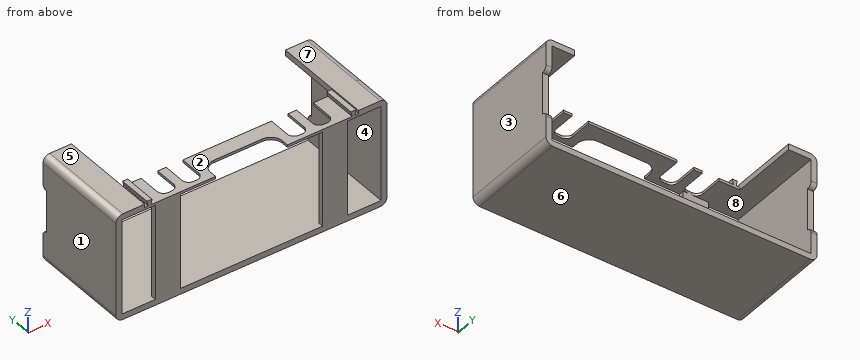
```python
from build123d import *

# Parameters (mm, degrees)
SKETCH1_W           = 81
SKETCH1_H           = 32
BOSS_EXTRUDE1_DEPTH = 10
SKETCH2_W           = 77.5
SKETCH2_H           = 28.5
CUT_EXTRUDE1_DEPTH  = 10
SKETCH3_W           = 7.5
SKETCH3_H           = 32
BOSS_EXTRUDE2_DEPTH = 1.5
SKETCH4_W           = 64
SKETCH4_H           = 1
CUT_EXTRUDE2_DEPTH  = 10
BOSS_EXTRUDE3_DEPTH = 10
BOSS_EXTRUDE4_DEPTH = 10
FILLET1_R           = 2
FILLET2_R           = 2
FILLET3_R           = 2
FILLET4_R           = 2
CUT_EXTRUDE3_DEPTH  = 0.75
SKETCH8_W           = 21.5
SKETCH8_H           = 5.5
CUT_EXTRUDE4_DEPTH  = 0.75
FILLET5_R           = 3.5
FILLET6_R           = 3.5
BOSS_EXTRUDE5_START = 20
BOSS_EXTRUDE5_DEPTH = 20
SKETCH10_W          = 1.75
SKETCH10_H          = 12.5
CUT_EXTRUDE5_DEPTH  = 1.5
FILLET7_R           = 1.5
FILLET8_R           = 1.5
FILLET10_R          = 1.5
FILLET11_R          = 1.5


with BuildPart() as part:
    # Sketch1 → Boss-Extrude1 (new body)
    with BuildSketch(Plane(origin=(0, 0, 0), x_dir=(1, 0, 0), z_dir=(0, 1, 0))):
        with Locations((-86.056207425, -60.23876691)):
            Rectangle(SKETCH1_W, SKETCH1_H)
    extrude(amount=BOSS_EXTRUDE1_DEPTH)

    # Sketch2 → Cut-Extrude1 (cut)
    with BuildSketch(Plane(origin=(0, 10, 0), x_dir=(1, 0, 0), z_dir=(0, 1, 0))):
        with Locations((-86.056207425, -60.23876691)):
            Rectangle(SKETCH2_W, SKETCH2_H)
    extrude(amount=-CUT_EXTRUDE1_DEPTH, mode=Mode.SUBTRACT)

    # Sketch3 → Boss-Extrude2 (add)
    with BuildSketch(Plane(origin=(0, 0, 0), x_dir=(-1, 0, 0), z_dir=(0, -1, 0))):
        with Locations((61.056207425, -60.23876691)):
            Rectangle(SKETCH3_W, SKETCH3_H)
        with Locations((111.056207425, -60.23876691)):
            Rectangle(SKETCH3_W, SKETCH3_H)
    extrude(amount=-BOSS_EXTRUDE2_DEPTH)

    # Sketch4 → Cut-Extrude2 (cut)
    with BuildSketch(Plane(origin=(0, 10, 0), x_dir=(1, 0, 0), z_dir=(0, 1, 0))):
        with Locations((-86.056207425, -75.73876691)):
            Rectangle(SKETCH4_W, SKETCH4_H)
    extrude(amount=-CUT_EXTRUDE2_DEPTH, mode=Mode.SUBTRACT)

    # Sketch5 → Boss-Extrude3 (add)
    with BuildSketch(Plane(origin=(0, 10, 0), x_dir=(1, 0, 0), z_dir=(0, 1, 0))):
        Polygon((-116.976207425, -75.23876691), (-117.306207425, -76.781751031), (-115.806207425, -76.781751031), (-116.146207425, -75.23876691), align=None)
    extrude(amount=-BOSS_EXTRUDE3_DEPTH)

    # Sketch6 → Boss-Extrude4 (add)
    with BuildSketch(Plane(origin=(0, 10, 0), x_dir=(1, 0, 0), z_dir=(0, 1, 0))):
        Polygon((-55.966207425, -75.23876691), (-56.306207425, -76.781751031), (-54.806207425, -76.781751031), (-55.136207425, -75.23876691), align=None)
    extrude(amount=-BOSS_EXTRUDE4_DEPTH)

    # Fillet1
    fillet1_edges = [part.edges().sort_by_distance(p)[0] for p in [
        (-126.556207425, 5, 76.23876691),
    ]]
    fillet(fillet1_edges, radius=FILLET1_R)

    # Fillet2
    fillet2_edges = [part.edges().sort_by_distance(p)[0] for p in [
        (-45.556207425, 5, 76.23876691),
    ]]
    fillet(fillet2_edges, radius=FILLET2_R)

    # Fillet3
    fillet3_edges = [part.edges().sort_by_distance(p)[0] for p in [
        (-45.556207425, 5, 44.23876691),
    ]]
    fillet(fillet3_edges, radius=FILLET3_R)

    # Fillet4
    fillet4_edges = [part.edges().sort_by_distance(p)[0] for p in [
        (-126.556207425, 5, 44.23876691),
    ]]
    fillet(fillet4_edges, radius=FILLET4_R)

    # Sketch7 → Cut-Extrude3 (cut)
    with BuildSketch(Plane.XY.offset(75.23876691)):
        with BuildLine():
            Line((-111.806207425, 10), (-106.806207425, 10))
            Line((-106.806207425, 10), (-106.806207425, 3.5))
            ThreePointArc((-106.806207425, 3.5), (-107.391993862, 2.085786438), (-108.806207425, 1.5))
            Line((-108.806207425, 1.5), (-109.806207425, 1.5))
            ThreePointArc((-109.806207425, 1.5), (-111.220420987, 2.085786438), (-111.806207425, 3.5))
            Line((-111.806207425, 3.5), (-111.806207425, 10))
        make_face()
        with BuildLine():
            Line((-65.306207425, 10), (-60.306207425, 10))
            Line((-60.306207425, 10), (-60.306207425, 3.5))
            ThreePointArc((-60.306207425, 3.5), (-60.891993862, 2.085786438), (-62.306207425, 1.5))
            Line((-62.306207425, 1.5), (-63.306207425, 1.5))
            ThreePointArc((-63.306207425, 1.5), (-64.720420987, 2.085786438), (-65.306207425, 3.5))
            Line((-65.306207425, 3.5), (-65.306207425, 10))
        make_face()
        with BuildLine():
            Line((-104.306207425, 10), (-99.306207425, 10))
            Line((-99.306207425, 10), (-99.306207425, 3.5))
            ThreePointArc((-99.306207425, 3.5), (-99.891993862, 2.085786438), (-101.306207425, 1.5))
            Line((-101.306207425, 1.5), (-102.306207425, 1.5))
            ThreePointArc((-102.306207425, 1.5), (-103.720420987, 2.085786438), (-104.306207425, 3.5))
            Line((-104.306207425, 3.5), (-104.306207425, 10))
        make_face()
        with BuildLine():
            Line((-72.806207425, 10), (-67.806207425, 10))
            Line((-67.806207425, 10), (-67.806207425, 3.5))
            ThreePointArc((-67.806207425, 3.5), (-68.391993862, 2.085786438), (-69.806207425, 1.5))
            Line((-69.806207425, 1.5), (-70.806207425, 1.5))
            ThreePointArc((-70.806207425, 1.5), (-72.220420987, 2.085786438), (-72.806207425, 3.5))
            Line((-72.806207425, 3.5), (-72.806207425, 10))
        make_face()
    extrude(amount=-CUT_EXTRUDE3_DEPTH, mode=Mode.SUBTRACT)

    # Sketch8 → Cut-Extrude4 (cut)
    with BuildSketch(Plane.XY.offset(75.23876691)):
        with Locations((-86.056207425, 2.75)):
            Rectangle(SKETCH8_W, SKETCH8_H)
    extrude(amount=-CUT_EXTRUDE4_DEPTH, mode=Mode.SUBTRACT)

    # Fillet5
    fillet5_edges = [part.edges().sort_by_distance(p)[0] for p in [
        (-96.806207425, 5.5, 74.86376691),
    ]]
    fillet(fillet5_edges, radius=FILLET5_R)

    # Fillet6
    fillet6_edges = [part.edges().sort_by_distance(p)[0] for p in [
        (-75.306207425, 5.5, 74.86376691),
    ]]
    fillet(fillet6_edges, radius=FILLET6_R)

    # Sketch9 → Boss-Extrude5 (add)
    with BuildSketch(Plane(origin=(0, 10, 0), x_dir=(1, 0, 0), z_dir=(0, 1, 0)).offset(BOSS_EXTRUDE5_START)):
        with BuildLine():
            Line((-47.556207425, -44.23876691), (-124.556207425, -44.23876691))
            ThreePointArc((-124.556207425, -44.23876691), (-125.970420987, -44.824553347), (-126.556207425, -46.23876691))
            Line((-126.556207425, -46.23876691), (-126.556207425, -74.23876691))
            ThreePointArc((-126.556207425, -74.23876691), (-125.970420987, -75.652980472), (-124.556207425, -76.23876691))
            Line((-124.556207425, -76.23876691), (-118.056207425, -76.23876691))
            Line((-118.056207425, -76.23876691), (-118.056207425, -75.23876691))
            Line((-118.056207425, -75.23876691), (-118.056207425, -74.48876691))
            Line((-118.056207425, -74.48876691), (-124.806207425, -74.48876691))
            Line((-124.806207425, -74.48876691), (-124.806207425, -45.98876691))
            Line((-124.806207425, -45.98876691), (-47.306207425, -45.98876691))
            Line((-47.306207425, -45.98876691), (-47.306207425, -74.48876691))
            Line((-47.306207425, -74.48876691), (-54.056207425, -74.48876691))
            Line((-54.056207425, -74.48876691), (-54.056207425, -75.23876691))
            Line((-54.056207425, -75.23876691), (-54.056207425, -76.23876691))
            Line((-54.056207425, -76.23876691), (-47.556207425, -76.23876691))
            ThreePointArc((-47.556207425, -76.23876691), (-46.141993862, -75.652980472), (-45.556207425, -74.23876691))
            Line((-45.556207425, -74.23876691), (-45.556207425, -46.23876691))
            ThreePointArc((-45.556207425, -46.23876691), (-46.141993862, -44.824553347), (-47.556207425, -44.23876691))
        make_face()
    extrude(amount=-BOSS_EXTRUDE5_DEPTH)

    # Sketch10 → Cut-Extrude5 (cut)
    with BuildSketch(Plane(origin=(0, 30, 0), x_dir=(1, 0, 0), z_dir=(0, 1, 0))):
        with Locations((-46.431207425, -60.23876691)):
            Rectangle(SKETCH10_W, SKETCH10_H)
        with Locations((-125.681207425, -60.23876691)):
            Rectangle(SKETCH10_W, SKETCH10_H)
    extrude(amount=-CUT_EXTRUDE5_DEPTH, mode=Mode.SUBTRACT)

    # Fillet7
    fillet7_edges = [part.edges().sort_by_distance(p)[0] for p in [
        (-125.681207425, 30, 66.48876691),
    ]]
    fillet(fillet7_edges, radius=FILLET7_R - 0.0001)  # a hair under: the kernel refuses the full size

    # Fillet8
    fillet8_edges = [part.edges().sort_by_distance(p)[0] for p in [
        (-125.681207425, 30, 53.98876691),
    ]]
    fillet(fillet8_edges, radius=FILLET8_R - 0.0001)  # a hair under: the kernel refuses the full size

    # Fillet10
    fillet10_edges = [part.edges().sort_by_distance(p)[0] for p in [
        (-46.431207425, 30, 53.98876691),
    ]]
    fillet(fillet10_edges, radius=FILLET10_R - 0.0001)  # a hair under: the kernel refuses the full size

    # Fillet11
    fillet11_edges = [part.edges().sort_by_distance(p)[0] for p in [
        (-46.431207425, 30, 66.48876691),
    ]]
    fillet(fillet11_edges, radius=FILLET11_R - 0.0001)  # a hair under: the kernel refuses the full size


solid = part.part
```
Geometry: final body of the model. Coordinates: model frame, mm. Face numbers are marked on the shaded views. A direction names the side the tool comes from. Round coordinates to 2 decimals unless told otherwise and drop trailing zeros. Write each loop counter-clockwise with the first axis right and the second up, starting at its lowest first coordinate (ties: lowest second). Pieces come first, ordered by that corner, then holes.
Item 1: Section query C-C (y = 25.75). Return loops of the section in (x, z).
Item 2: Section query A-A (z = 48). Return loops of the section in (x, y), plus the area to 4 significant figures.
Item 3: Set-up query: the marked faces 4, 5, 6, 7 and 8. Return all of +Z, -Z, +X, -X, +Y, -Y with unobstructed straight access to the full face (end or side cutting, diameter ignored); none if empty.
Item 4: Section query D-D (z = 59.5). Return loops of the section in (x, y), plus the area to 3 significant figures.
Item 5: Mould query, pull axis X, two halves, no side actions, for the marked faces 1, 2 and 3. Classes: +X half, -X half, draft (parallel to the pull), parting line (faces both ways), or undercut.
Item 6: Section query B-B (x = -51). Return loops of the section in (y, z).
Item 7: Material intervals for L1, parallel to X at y = 17.5, z = 71; L2, parallel to Z at x = -73.5, y = 5; L3, parallel to Z at x = -119, y = 15.25, sorted ascending.
Item 8: Pin query (flat end, axial travel): P1, Ø2, axis at x = -106, z = 55.5, coming from the -Y side; P2, Ø1.4, axis at x = -125.5, z = 59.5, coming from the +Y side; P3, Ø0.8, axis at y = 6.5, z = 75, coming from the -X side; P4, Ø1.8, axis at x = -114.5, z = 75, coming from the +Y side. Return the tip coordinate at first contact, or that it passes through.
Completed:
1. outline: (-126.56, 46.24) arc R2 ccw to (-124.56, 44.24) - (-47.56, 44.24) arc R2 ccw to (-45.56, 46.24) - (-45.56, 74.24) arc R2 ccw to (-47.56, 76.24) - (-54.06, 76.24) - (-54.06, 74.49) - (-47.31, 74.49) - (-47.31, 45.99) - (-124.81, 45.99) - (-124.81, 74.49) - (-118.06, 74.49) - (-118.06, 76.24) - (-124.56, 76.24) arc R2 ccw to (-126.56, 74.24) - close
2. outline: (-126.56, 0) - (-124.81, 0) - (-124.81, 30) - (-126.56, 30) - close; (-114.81, 0) - (-107.31, 0) - (-107.31, 1.5) - (-114.81, 1.5) - close; (-64.81, 0) - (-57.31, 0) - (-57.31, 1.5) - (-64.81, 1.5) - close; (-47.31, 0) - (-45.56, 0) - (-45.56, 30) - (-47.31, 30) - close
2. area: 127.5 mm2
3. face 4: +Y, -Y
3. face 5: +Z, -X, +Y, -Y
3. face 6: -Z, +X, -X, +Y, -Y
3. face 7: +Z, +X, +Y, -Y
3. face 8: +Y
4. outline: (-126.56, 0) - (-124.81, 0) - (-124.81, 28.5) - (-126.56, 28.5) - close; (-114.81, 0) - (-107.31, 0) - (-107.31, 1.5) - (-114.81, 1.5) - close; (-64.81, 0) - (-57.31, 0) - (-57.31, 1.5) - (-64.81, 1.5) - close; (-47.31, 0) - (-45.56, 0) - (-45.56, 28.5) - (-47.31, 28.5) - close
4. area: 122 mm2
5. face 1: -X half
5. face 2: undercut
5. face 3: +X half
6. outline: (0, 44.24) - (30, 44.24) - (30, 45.99) - (0, 45.99) - close; (0, 74.49) - (30, 74.49) - (30, 76.24) - (0, 76.24) - close
7. L1: x = -126.56 to -124.81, -47.31 to -45.56
7. L2: z = 44.24 to 45.99, 74.49 to 75.24
7. L3: z = 44.24 to 45.99, 74.49 to 76.24
8. P1: passes through
8. P2: stops at y = 28.5
8. P3: stops at x = -126.52
8. P4: stops at y = 10
